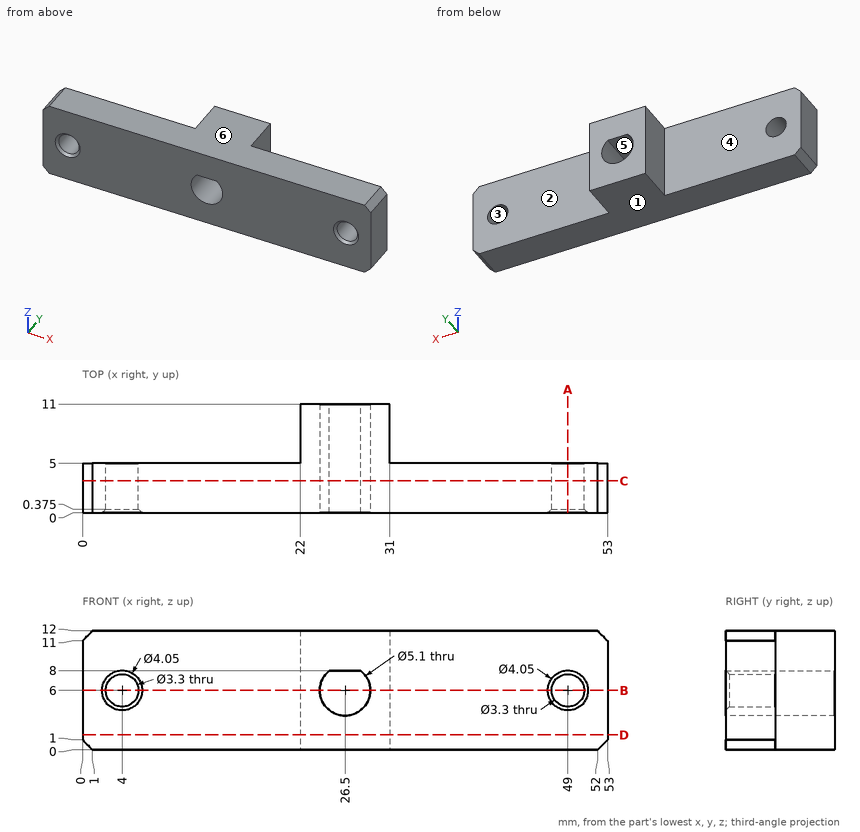
Design review of the part shown in the three views and the two pictorial views. Dimensions are in mm from the part's minimum x, y and z. A direction names the side the tool comes from. Give positions to 0.01 mm unless a question says otherwise; leave off trailing zeros. Loops run counter-clockwise (first coordinate to the right, second up) from the corner with the lowest first, then second, coordinate; pieces in that order, holes last. Notation, with made-up numbers: M 9.25,78.25 L 34.25,78.25 A14 ccw 34.25,105.25 Z; hole C 58,27.25 d8. An arc over 180 degrees is marked long. Answer as a JSON object with one key per item and string values. Group by question number.
Q1. Add section D-D on z = 1.5. Give the boundary of the cut face in (x, y), and give its area (3 significant figures).
Q2. Insertion check: P1, Ø5, axis at y = 8, z = 3.5, coming from the -X side; P2, Ø4.5, axis at x = 49, z = 6, coming from the +Y side; P3, Ø3, axis at y = 7.5, z = 3.5, coming from the +X side. Each pin has a flat end and moves straight along its axis. Give the tip position at first contact, or say it passes through.
Q3. Add section B-B on z = 6. Give the boundary of the cut face in (x, y) (3 decimals), and give its area (3 significant figures).
Q4. Add section A-A on x = 49. Give the boundary of the cut face in (y, z) (3 decimals), and give its area (3 significant figures).
Q5. Add section C-C on y = 3.25. Give the boundary of the cut face in (x, z).
Q6. For probe 1 along X at (y, z) = (4.75, 7); probe 2 along Z at (x, y) = (49, 2.5); probe 3 along X at (y, z) = (5.75, 6), list the stretches that pass through material, from the lowest coordinate up. Write a range as [from, to].
Q7. Tool access review of the marked faces 4, 5 and 6: name each direction out of +Z, -Z, +X, -X, +Y, -Y from which nothing blocks a thin tool from reaching the whole face with its end or side.
Q8. Mouldability with a two-part tool opening along Z and no side actions: class the marked faces 1, 2 and 3 as +Z half, -Z half, draft (parallel to the pull), parting line (faces both ways), or undercut.
Checked values:
{
 "1": {"outline": "M 0,0 L 53,0 L 53,5 L 31,5 L 31,11 L 22,11 L 22,5 L 0,5 Z", "area": "319 mm²"},
 "2": {"P1": "x = 22", "P2": "y = 5", "P3": "x = 31"},
 "3": {"outline": "M 0,0 L 1.975,0 L 2.35,0.375 L 2.35,5 L 0,5 Z; M 5.65,0.375 L 6.025,0 L 23.95,0 L 23.95,11 L 22,11 L 22,5 L 5.65,5 Z; M 29.05,0 L 46.975,0 L 47.35,0.375 L 47.35,5 L 31,5 L 31,11 L 29.05,11 Z; M 50.65,0.375 L 51.025,0 L 53,0 L 53,5 L 50.65,5 Z", "area": "230 mm²"},
 "4": {"outline": "M 0,0 L 5,0 L 5,4.35 L 0.375,4.35 L 0,3.975 Z; M 0,8.025 L 0.375,7.65 L 5,7.65 L 5,12 L 0,12 Z", "area": "43.4 mm²"},
 "5": {"outline": "M 0,1 L 1,0 L 52,0 L 53,1 L 53,11 L 52,12 L 1,12 L 0,11 Z; hole C 4,6 d3.3; hole M 24.92,8 A2.55 ccw long 28.08,8 Z; hole C 49,6 d3.3"},
 "6": {"probe 1": "[0, 2.69], [5.31, 24.15], [28.85, 47.69], [50.31, 53]", "probe 2": "[0, 4.35], [7.65, 12]", "probe 3": "[22, 23.95], [29.05, 31]"},
 "7": {"face 4": "+Z, -Z, -X, +Y", "face 5": "+Y, -Y", "face 6": "+Z, +X, -X, +Y, -Y"},
 "8": {"face 1": "-Z half", "face 2": "draft", "face 3": "undercut"}
}
